Input: part model. Units: mm. Frame: model coordinates. Face numbers are marked on the shaded views. A direction names the side the tool comes from. Round coordinates to 2 decimals unless told otherwise and drop trailing zeros. Loops run counter-clockwise (first coordinate to the right, second up) from the corner with the lowest first, then second, coordinate; pieces in that order, holes last. Notation, with made-up numbers: (36, 56) -> (69, 56) arc R38 cw to (69, 95) -> close; hole circle Ø5 at (-2.5, 19). An arc over 180 degrees is marked (long way). Answer in a Markdown table with one row per item. Add a question column.
Q1. Section C-C, the plane y = -3. Output: boundary loops of the cut face in (x, z), and give its area (3 significant figures).
Q2. Section D-D, the plane x = -15. Output: boundary loops of the cut face in (y, z), and give its area (3 significant figures).
Q3. Mould query, pull axis X, two halves, no side actions, for the marked faces 6, 7, 8 and 9. Classes: pulls with the +X half, pulls with the -X half, needs draft (parallel to the pull), parting line crosses it, or undercut.
Q4. Section A-A, the plane z = -56.5. Output: boundary loops of the cut face in (x, y), and give its area (3 significant figures).
Q5. Ray query, L1, parallel to Z at x = 0, y = -9; L2, parallel to Y at x = 30, z = -33; L3, parallel to Z at x = -10, y = -8.5. Return the intervals inside material, ascending. Write a range as from..to.
Q6. Section B-B, the plane x = 0. Output: boundary loops of the cut face in (y, z).
Q7. Reachability of the marked faces 1, 2, 3, 4 and 5 from +Z, -Z, +X, -X, +Y, -Y: full face, straight path, thin tool, end or side. Return the list, or none.
Q8. Pin query (flat end, axial travel): pin 1 (15 mm diameter, centred on y = -9.5, z = 17.5, fed in from -X); pin 2 (24 mm diameter, centred on x = 0, z = 2.28, fed in from +Y); pin 3 (5.5 mm diameter, centred on x = 11, y = -5.5, fed in from -Z). Return the tip coordinate at first contact, or that it passes through.
```python
from build123d import *

# Parameters (mm, degrees)
F1_DEPTH = 19.05
F2_R     = 9.20198
F3_DEPTH = 19.05
F5_DEPTH = 19.05


with BuildPart() as f1:
    # F0 (on Front) → F1 (new body)
    with BuildSketch(Plane.XZ):
        Polygon((38.1, 48.757284), (-38.1, 48.757284), (-38.1, -65.542716), (-25.4, -65.542716), (-25.4, -27.442716), (25.4, -27.442716), (25.4, -65.542716), (38.1, -65.542716), align=None)
    extrude(amount=F1_DEPTH)

    # F2 (on face) → F3 (cut)
    with BuildSketch(Plane.XZ.offset(19.05)):
        with Locations((0, 2.275284)):
            Circle(F2_R)
    extrude(amount=-F3_DEPTH, mode=Mode.SUBTRACT)

    # F4 (on face) → F5 (join)
    with BuildSketch(Plane.XY.offset(48.757284)):
        Polygon((-38.222246, 44.45), (-38.222246, -19.05), (38.1, -19.05), (38.1, 19.05), (12.577754, 44.45), align=None)
    extrude(amount=F5_DEPTH)


solid = f1.part
```
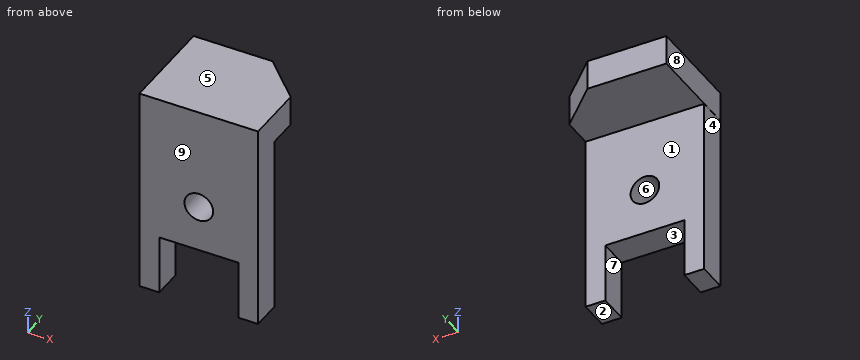
Answer block:
| question | item | result |
|---|---|---|
| 1 | outline | (-38.22, 48.76) -> (-38.1, 48.76) -> (-38.1, -65.54) -> (-25.4, -65.54) -> (-25.4, -27.44) -> (25.4, -27.44) -> (25.4, -65.54) -> (38.1, -65.54) -> (38.1, 67.81) -> (-38.22, 67.81) -> close; hole circle Ø18.4 at (0, 2.28) |
| 1 | area | 7,960 mm^2 |
| 2 | outline | (-19.05, -27.44) -> (0, -27.44) -> (0, 48.76) -> (44.45, 48.76) -> (44.45, 67.81) -> (-19.05, 67.81) -> close |
| 2 | area | 2,660 mm^2 |
| 3 | face 6 | undercut |
| 3 | face 7 | undercut |
| 3 | face 8 | pulls with the -X half |
| 3 | face 9 | needs draft |
| 4 | outline | (-38.1, -19.05) -> (-25.4, -19.05) -> (-25.4, 0) -> (-38.1, 0) -> close; (25.4, -19.05) -> (38.1, -19.05) -> (38.1, 0) -> (25.4, 0) -> close |
| 4 | area | 484 mm^2 |
| 5 | L1 | -27.44..-6.93, 11.48..67.81 |
| 5 | L2 | -19.05..0 |
| 5 | L3 | -27.44..67.81 |
| 6 | outline | (-19.05, -27.44) -> (0, -27.44) -> (0, -6.93) -> (-19.05, -6.93) -> close; (-19.05, 11.48) -> (0, 11.48) -> (0, 48.76) -> (44.45, 48.76) -> (44.45, 67.81) -> (-19.05, 67.81) -> close |
| 7 | face 1 | -Z, +X, -X, +Y |
| 7 | face 2 | -Z, +X, -X, +Y, -Y |
| 7 | face 3 | -Z, +Y, -Y |
| 7 | face 4 | -Z, -X, +Y, -Y |
| 7 | face 5 | +Z, +X, -X, +Y, -Y |
| 8 | pin 1 | x = -38.1 |
| 8 | pin 2 | y = 0 |
| 8 | pin 3 | z = -27.44 |
